Could you check a few things on this model? Use its own coordinates, in mm. Face numbers are marked on the shaded views. A direction names the side the tool comes from. Round coordinates to 2 decimals unless told otherwise and drop trailing zeros. Write each loop counter-clockwise with the first axis right and the second up, starting at its lowest first coordinate (ties: lowest second). Pieces come first, ordered by that corner, then holes. Notation, with made-up numbers: (-4.5, 89.5) -> (12.5, 89.5) arc R22 cw to (12.5, 122.5) -> close; hole circle Ø9 at (-8, 55). An arc over 180 degrees is marked (long way). Answer in a Markdown table with one row per item. Add a question column.
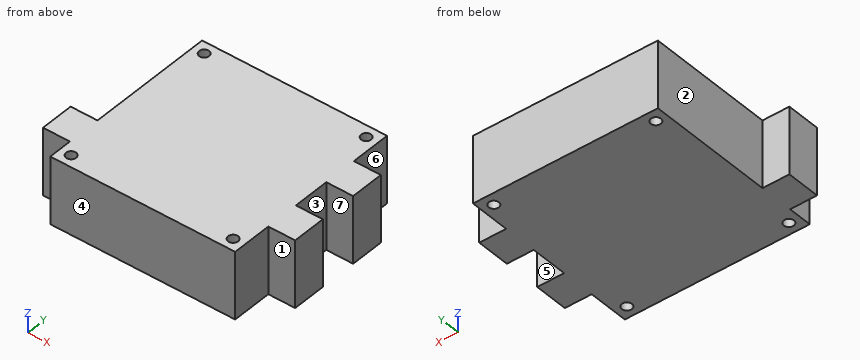
```python
from build123d import *

# Parameters (mm, degrees)
SKETCH_1_R      = 1.5
EXTRUDE_1_DEPTH = 20


with BuildPart() as part:
    # 草图1 → 凸台-拉伸1 (new body)
    with BuildSketch(Plane.XY):
        Polygon((-27.5, -20.402404897), (-35.5, -20.402404897), (-35.5, -10.402404897), (-27.5, -10.402404897), (-27.5, 27.5), (27.5, 27.5), (27.5, 15.5), (35.5, 15.5), (35.5, 5.5), (27.5, 5.5), (27.5, -5.5), (35.5, -5.5), (35.5, -15.5), (27.5, -15.5), (27.5, -27.5), (-27.5, -27.5), align=None)
        with Locations((-24.1, 24.1)):
            Circle(SKETCH_1_R, mode=Mode.SUBTRACT)
        with Locations((24.1, 24.1)):
            Circle(SKETCH_1_R, mode=Mode.SUBTRACT)
        with Locations((-24.1, -24.1)):
            Circle(SKETCH_1_R, mode=Mode.SUBTRACT)
        with Locations((24.1, -24.1)):
            Circle(SKETCH_1_R, mode=Mode.SUBTRACT)
    extrude(amount=EXTRUDE_1_DEPTH)


solid = part.part
```
(1) Suppose I cut it at D-D, the plane x = -30. Please give me the cut outline in (y, z), then the cut area to 3 significant figures.
(2) I need wall thicknesses on L1, parallel to X at y = 24, z = 3.25; L2, parallel to Y at x = 29, z = 2.75. Which ranges of each line are inside material? Lowest first, please.
(3) Suppose I cut it at C-C, the plane z = 10. Please give me the cut outline in (x, y).
(4) On a 3-axis mill with a long thin cutter (end or side, diameter ignored), from which of +Z, -Z, +X, -X, +Y, -Y can I reach the whole of each face in a straight line? I mean the marked faces 1, 2 and 3. Say none if no direction works.
(5) If we mould it in two halves opening along Y, with no side actions, what happens to the marked faces 4, 5, 6 and 7? For each: pulls with the +Y half, pulls with the -Y half, needs draft (parallel to the pull), parting line crosses it, or undercut.
(6) Suppose I cut it at A-A, the plane y = 24.1. Please give me the cut outline in (x, z).
(7) For P1, Ø2, axis at y = 21, z = 7, coming from the +X side; P2, Ø6.5, axis at x = 32, z = 13.5, coming from the +Y side; P3, Ø2, axis at y = 21.5, z = 8, coming from the -X side, each with a flat end and sliding along its axis, tell me the tip position at first contact or that it passes through.
Response:
| question | item | result |
|---|---|---|
| 1 | outline | (-20.4, 0) -> (-10.4, 0) -> (-10.4, 20) -> (-20.4, 20) -> close |
| 1 | area | 200 mm² |
| 2 | L1 | -27.5 to -25.6, -22.6 to 22.6, 25.6 to 27.5 |
| 2 | L2 | -15.5 to -5.5, 5.5 to 15.5 |
| 3 | outline | (-35.5, -20.4) -> (-27.5, -20.4) -> (-27.5, -27.5) -> (27.5, -27.5) -> (27.5, -15.5) -> (35.5, -15.5) -> (35.5, -5.5) -> (27.5, -5.5) -> (27.5, 5.5) -> (35.5, 5.5) -> (35.5, 15.5) -> (27.5, 15.5) -> (27.5, 27.5) -> (-27.5, 27.5) -> (-27.5, -10.4) -> (-35.5, -10.4) -> close; hole circle Ø3 at (-24.1, -24.1); hole circle Ø3 at (-24.1, 24.1); hole circle Ø3 at (24.1, -24.1); hole circle Ø3 at (24.1, 24.1) |
| 4 | face 1 | +Z, -Z, +X, -Y |
| 4 | face 2 | +Z, -Z, -X, +Y |
| 4 | face 3 | +Z, -Z, +X |
| 5 | face 4 | pulls with the -Y half |
| 5 | face 5 | undercut |
| 5 | face 6 | needs draft |
| 5 | face 7 | undercut |
| 6 | outline | (-27.5, 0) -> (-25.6, 0) -> (-25.6, 20) -> (-27.5, 20) -> close; (-22.6, 0) -> (22.6, 0) -> (22.6, 20) -> (-22.6, 20) -> close; (25.6, 0) -> (27.5, 0) -> (27.5, 20) -> (25.6, 20) -> close |
| 7 | P1 | x = 27.5 |
| 7 | P2 | y = 15.5 |
| 7 | P3 | x = -27.5 |
